from build123d import *

# Parameters (mm, degrees)
SKETCH1_W                     = 21
SKETCH1_H                     = 21
BOSS_EXTRUDE1_DEPTH           = 1.85
SKETCH2_W                     = 9
SKETCH2_H                     = 9
BOSS_EXTRUDE2_DEPTH           = 2
SKETCH3_R                     = 1.875
CUT_EXTRUDE1_DEPTH            = 1.85
SKETCH4_W                     = 2
SKETCH4_H                     = 1
SKETCH4_W_2                   = 1
SKETCH4_H_2                   = 2
BOSS_EXTRUDE3_DEPTH           = 0.5
SKETCH5_R                     = 0.75
BOSS_EXTRUDE4_DEPTH           = 2
BOSS_EXTRUDE4_DRAFT           = -10
BOSS_EXTRUDE4_PROFILE_2_DEPTH = 2
BOSS_EXTRUDE4_PROFILE_2_DRAFT = -10
BOSS_EXTRUDE4_PROFILE_3_DEPTH = 2
BOSS_EXTRUDE4_PROFILE_3_DRAFT = -10
BOSS_EXTRUDE4_PROFILE_4_DEPTH = 2
BOSS_EXTRUDE4_PROFILE_4_DRAFT = -10
BOSS_EXTRUDE5_DEPTH           = 1.5
SKETCH7_R                     = 0.25
BOSS_EXTRUDE6_DEPTH           = 11.5


with BuildPart() as part:
    # Sketch1 → Boss-Extrude1 (new body)
    with BuildSketch(Plane(origin=(0, 0, 0), x_dir=(1, 0, 0), z_dir=(0, 1, 0))):
        Rectangle(SKETCH1_W, SKETCH1_H)
    extrude(amount=BOSS_EXTRUDE1_DEPTH)

    # Sketch2 → Boss-Extrude2 (add)
    with BuildSketch(Plane(origin=(0, 1.85, 0), x_dir=(1, 0, 0), z_dir=(0, 1, 0))):
        with Locations((1.5, -0.5)):
            Rectangle(SKETCH2_W, SKETCH2_H)
    extrude(amount=BOSS_EXTRUDE2_DEPTH)

    # Sketch3 → Cut-Extrude1 (cut)
    with BuildSketch(Plane(origin=(0, 1.85, 0), x_dir=(1, 0, 0), z_dir=(0, 1, 0))):
        with Locations(Location((7.625, -7.625, 0), (0, 0, 270))):
            Circle(SKETCH3_R)
        with Locations(Location((-7.625, 7.625, 0), (0, 0, 270))):
            Circle(SKETCH3_R)
    extrude(amount=-CUT_EXTRUDE1_DEPTH, mode=Mode.SUBTRACT)

    # Sketch4 → Boss-Extrude3 (add)
    with BuildSketch(Plane(origin=(0, 1.85, 0), x_dir=(1, 0, 0), z_dir=(0, 1, 0))):
        with Locations((1.5, 9)):
            Rectangle(SKETCH4_W, SKETCH4_H)
        with Locations((1.5, 7)):
            Rectangle(SKETCH4_W, SKETCH4_H)
        with Locations((8, 6.5)):
            Rectangle(SKETCH4_W, SKETCH4_H)
        with Locations((7.5, 2)):
            Rectangle(SKETCH4_W_2, SKETCH4_H_2)
        with Locations((9, 2)):
            Rectangle(SKETCH4_W_2, SKETCH4_H_2)
    extrude(amount=BOSS_EXTRUDE3_DEPTH)


with BuildPart() as boss_extrude4_tool:
    # Sketch5 → Boss-Extrude4 (with draft: the straight prism first)
    with BuildSketch(Plane(origin=(0, 0, 0), x_dir=(1, 0, 0), z_dir=(0, 1, 0))):
        with Locations((-9.25, 2.75)):
            Circle(SKETCH5_R)
    extrude(amount=-BOSS_EXTRUDE4_DEPTH)
    # Boss-Extrude4: the draft: its side faces are tilted about the plane it starts from
    boss_extrude4_sides = [boss_extrude4_tool.faces().sort_by_distance(p)[0] for p in [
        (-10, -1, -2.75),
    ]]
    draft(boss_extrude4_sides, Plane(origin=(0, 0, 0), x_dir=(1, 0, 0), z_dir=(0, 1, 0)), BOSS_EXTRUDE4_DRAFT)


with BuildPart() as part_1:
    add(part.part)

    # Boss-Extrude4: add boss_extrude4_tool
    add(boss_extrude4_tool.part)


with BuildPart() as boss_extrude4_profile_2_tool:
    # Sketch5 → Boss-Extrude4 profile 2 (with draft: the straight prism first)
    with BuildSketch(Plane(origin=(0, 0, 0), x_dir=(1, 0, 0), z_dir=(0, 1, 0))):
        with Locations((-9.25, 0.25)):
            Circle(SKETCH5_R)
    extrude(amount=-BOSS_EXTRUDE4_PROFILE_2_DEPTH)
    # Boss-Extrude4 profile 2: the draft: its side faces are tilted about the plane it starts from
    boss_extrude4_profile_2_sides = [boss_extrude4_profile_2_tool.faces().sort_by_distance(p)[0] for p in [
        (-10, -1, -0.25),
    ]]
    draft(boss_extrude4_profile_2_sides, Plane(origin=(0, 0, 0), x_dir=(1, 0, 0), z_dir=(0, 1, 0)), BOSS_EXTRUDE4_PROFILE_2_DRAFT)


with BuildPart() as part_2:
    add(part_1.part)

    # Boss-Extrude4 profile 2: add boss_extrude4_profile_2_tool
    add(boss_extrude4_profile_2_tool.part)


with BuildPart() as boss_extrude4_profile_3_tool:
    # Sketch5 → Boss-Extrude4 profile 3 (with draft: the straight prism first)
    with BuildSketch(Plane(origin=(0, 0, 0), x_dir=(1, 0, 0), z_dir=(0, 1, 0))):
        with Locations((-9.25, -2.25)):
            Circle(SKETCH5_R)
    extrude(amount=-BOSS_EXTRUDE4_PROFILE_3_DEPTH)
    # Boss-Extrude4 profile 3: the draft: its side faces are tilted about the plane it starts from
    boss_extrude4_profile_3_sides = [boss_extrude4_profile_3_tool.faces().sort_by_distance(p)[0] for p in [
        (-10, -1, 2.25),
    ]]
    draft(boss_extrude4_profile_3_sides, Plane(origin=(0, 0, 0), x_dir=(1, 0, 0), z_dir=(0, 1, 0)), BOSS_EXTRUDE4_PROFILE_3_DRAFT)


with BuildPart() as part_3:
    add(part_2.part)

    # Boss-Extrude4 profile 3: add boss_extrude4_profile_3_tool
    add(boss_extrude4_profile_3_tool.part)


with BuildPart() as boss_extrude4_profile_4_tool:
    # Sketch5 → Boss-Extrude4 profile 4 (with draft: the straight prism first)
    with BuildSketch(Plane(origin=(0, 0, 0), x_dir=(1, 0, 0), z_dir=(0, 1, 0))):
        with Locations((-9.25, -4.75)):
            Circle(SKETCH5_R)
    extrude(amount=-BOSS_EXTRUDE4_PROFILE_4_DEPTH)
    # Boss-Extrude4 profile 4: the draft: its side faces are tilted about the plane it starts from
    boss_extrude4_profile_4_sides = [boss_extrude4_profile_4_tool.faces().sort_by_distance(p)[0] for p in [
        (-10, -1, 4.75),
    ]]
    draft(boss_extrude4_profile_4_sides, Plane(origin=(0, 0, 0), x_dir=(1, 0, 0), z_dir=(0, 1, 0)), BOSS_EXTRUDE4_PROFILE_4_DRAFT)


with BuildPart() as part_4:
    add(part_3.part)

    # Boss-Extrude4 profile 4: add boss_extrude4_profile_4_tool
    add(boss_extrude4_profile_4_tool.part)

    # Sketch6 → Boss-Extrude5 (add)
    with BuildSketch(Plane.XZ.offset(-1.85)):
        with BuildLine():
            Line((-10, -1.25), (-10, -1.75))
            ThreePointArc((-10, -1.75), (-9.25, -4), (-8.5, -1.75))
            Line((-8.5, -1.75), (-8.5, -1.25))
            ThreePointArc((-8.5, -1.25), (-8, -0.25), (-8.5, 0.75))
            Line((-8.5, 0.75), (-8.5, 1.25))
            ThreePointArc((-8.5, 1.25), (-8, 2.25), (-8.5, 3.25))
            Line((-8.5, 3.25), (-8.5, 3.75))
            ThreePointArc((-8.5, 3.75), (-9.25, 6), (-10, 3.75))
            Line((-10, 3.75), (-10, 3.25))
            ThreePointArc((-10, 3.25), (-10.5, 2.25), (-10, 1.25))
            Line((-10, 1.25), (-10, 0.75))
            ThreePointArc((-10, 0.75), (-10.5, -0.25), (-10, -1.25))
        make_face()
    extrude(amount=-BOSS_EXTRUDE5_DEPTH)

    # Sketch7 → Boss-Extrude6 (add)
    with BuildSketch(Plane(origin=(0, 3.35, 0), x_dir=(-1, 0, 0), z_dir=(0, 1, 0))):
        with Locations(Location((9.25, -2.75, 0), (0, 0, 270))):
            Circle(SKETCH7_R)
        with Locations(Location((9.25, -0.25, 0), (0, 0, 270))):
            Circle(SKETCH7_R)
        with Locations(Location((9.25, 2.25, 0), (0, 0, 270))):
            Circle(SKETCH7_R)
        with Locations(Location((9.25, 4.75, 0), (0, 0, 270))):
            Circle(SKETCH7_R)
    extrude(amount=BOSS_EXTRUDE6_DEPTH)


solid = part_4.part
Check sheet for the modelled part. Datum: model origin and axes. Units: mm. A direction names the side the tool comes from. Give positions to 0.01 mm unless a question says otherwise; leave off trailing zeros. Loops run counter-clockwise (first coordinate to the right, second up) from the corner with the lowest first, then second, coordinate; pieces in that order, holes last. Notation, with made-up numbers: M 82,-13 L 123,-13 A35 cw 123,19 Z; hole C 54.25,-1 d5. An arc over 180 degrees is marked long. Answer as a JSON object with one key per item and string values. Group by question number.
Q1. Access from +Z, -Z, +X, -X, +Y, -Y to the whole of each face (thin tool, end or side, straight path). Record for faces 1 (the cylindrical face through (-10.5, 2.6, -0.2)), 2 (the flat face through (-3, 3, 1)), 3 (the cylindrical face through (-9.2, 2.6, 6)).
Q2. Cross-section at A-A on y = 7.5. Record the cut outline in (x, z).
Q3. Release check for a two-part mould opening along Z. For faces 4 (the flat face through (1, 3, 5)), 5 (the cylindrical face through (-9.455, 0.938, -8.031)), 6 (the flat face through (1, 3.85, 0)) record: released by +Z, released by -Z, zero draft, split by the parting line, or undercut.
Q4. Go/stop test with flat-tipped pins: P1, Ø1.6, axis at y = 3, z = -1, coming from the +X side; P2, Ø5, axis at y = 7, z = 2, coming from the -X side; P3, Ø10, axis at y = 3.5, z = 3, coming from the +X side; P4, Ø1.5, axis at x = 2.5, z = -1.5, coming from the +Y side. Record where each tip stops, or that it passes through.
Q5. Material ranges on line 1 along Y through (x, z) = (-4.5, 5); line 2 along Y through (x, z) = (4.75, -1.5); line 3 along X through (y, z) = (7, 4.75), recorded low to high. Write a range as [from, to].
Q6. Cross-section at B-B on z = -9. Record the cut outline in (x, y).
Evaluation:
{
 "1": {"face 1": "-X, +Y", "face 2": "+Z, -Z, +Y", "face 3": "+Y"},
 "2": {"outline": "C -9.25,-2.75 d0.5; C -9.25,-0.25 d0.5; C -9.25,2.25 d0.5; C -9.25,4.75 d0.5"},
 "3": {"face 4": "released by +Z", "face 5": "undercut", "face 6": "zero draft"},
 "4": {"P1": "stops at x = 9.5", "P2": "stops at x = -9.5", "P3": "stops at x = 10.5", "P4": "stops at y = 3.85"},
 "5": {"line 1": "y = [0, 1.85]", "line 2": "y = [0, 3.85]", "line 3": "x = [-9.5, -9]"},
 "6": {"outline": "M -10.5,0 L -8.9,0 L -8.9,1.85 L -10.5,1.85 Z; M -6.35,0 L 10.5,0 L 10.5,1.85 L 2.5,1.85 L 2.5,2.35 L 0.5,2.35 L 0.5,1.85 L -6.35,1.85 Z"}
}
